from build123d import *

# Parameters (mm, degrees)
SZKIC2_W                    = 70
SZKIC2_H                    = 50
DODANIE_WYCI_GNI_CIE1_DEPTH = 5
OTW_R_3_2_3_2_1_D           = 3.2
OTW_R_3_2_3_2_1_DEPTH       = 5
OTW_R_3_2_3_2_1_TIP         = 0.96137699
WYTNIJ_WYCI_GNI_CIE1_REACH  = 45.301
SZKIC7_R                    = 6
DODANIE_WYCI_GNI_CIE2_DEPTH = 5
SFAZOWANIE1_SIZE            = 2


with BuildPart() as part:
    # Szkic2 → Dodanie-wyciągnięcie1 (new body)
    with BuildSketch(Plane(origin=(0, 0, 0), x_dir=(1, 0, 0), z_dir=(0, 1, 0))):
        Rectangle(SZKIC2_W, SZKIC2_H)
    extrude(amount=DODANIE_WYCI_GNI_CIE1_DEPTH)

    # Otwór Ø3.2 (3.2)1
    with Locations(Plane(origin=(0, 5, 0), x_dir=(1, 0, 0), z_dir=(0, 1, 0))):
        with Locations((-7.75, -14.423393759), (7.75, -14.423393759), (15.5, -1), (7.75, 12.423393759), (-7.75, 12.423393759), (-15.5, -1)):
            Hole(OTW_R_3_2_3_2_1_D / 2, depth=OTW_R_3_2_3_2_1_DEPTH)
            with Locations((0, 0, -(OTW_R_3_2_3_2_1_DEPTH + OTW_R_3_2_3_2_1_TIP / 2))):  # 118° drill point
                Cone(0, OTW_R_3_2_3_2_1_D / 2, OTW_R_3_2_3_2_1_TIP, mode=Mode.SUBTRACT)

    # Szkic7 → Wytnij-wyciągnięcie1 (cut, up to next)
    with BuildSketch(Plane(origin=(0, 5, 0), x_dir=(1, 0, 0), z_dir=(0, 1, 0)), mode=Mode.PRIVATE) as wytnij_wyci_gni_cie1_sk1:
        with Locations(Location((0, 6, 0), (0, 0, 270))):
            Circle(SZKIC7_R)
    wytnij_wyci_gni_cie1_tool1 = extrude(wytnij_wyci_gni_cie1_sk1.sketch, amount=-WYTNIJ_WYCI_GNI_CIE1_REACH, mode=Mode.PRIVATE) & part.part
    add(wytnij_wyci_gni_cie1_tool1.solids().sort_by_distance((0, 5, -6))[0], mode=Mode.SUBTRACT)

    # Szkic8 → Dodanie-wyciągnięcie2 (add)
    with BuildSketch(Plane(origin=(0, 0, -25), x_dir=(-1, 0, 0), z_dir=(0, 0, -1))):
        Polygon((-35, 5), (-35, 55), (35, 55), (35, 5), (35, 0), (-35, 0), align=None)
    extrude(amount=DODANIE_WYCI_GNI_CIE2_DEPTH)

    # Sfazowanie1
    sfazowanie1_edges = [part.edges().sort_by_distance(p)[0] for p in [
        (0, 5, -25),
    ]]
    chamfer(sfazowanie1_edges, length=SFAZOWANIE1_SIZE)


solid = part.part
Input: part model. Units: mm. Frame: model coordinates. A direction names the side the tool comes from. Give positions to 0.01 mm unless a question says otherwise; leave off trailing zeros. Write each loop counter-clockwise with the first axis right and the second up, starting at its lowest first coordinate (ties: lowest second). Pieces come first, ordered by that corner, then holes. Notation, with made-up numbers: M -33,-14.5 L 17,-14.5 A18 ccw 17,13.5 Z; hole C -24.75,-2.5 d1. An arc over 180 degrees is marked long. Write item = value, one per line. Start each with the question number.
1) Draft query along Z for faces 3 (the flat face through (0, 2, 25)), 4 (the cylindrical face through (7.96, 2.46, -14.01)), 5 (the flat face through (35, 15, -27)). Return one class per face: +Z half, -Z half, draft (parallel to the pull), parting line (faces both ways), or undercut.
2) First-contact query: pin 1 Ø1.9 at (x, z) = (-7.75, -12.42) entering from +Y; pin 2 Ø14.5 at (x, z) = (-16, 3) entering from +Y. Flat tips, straight axial feed; report the tip coordinate or a pass-through.
3) Cut plane C-C on x = -15.5. Return the cut outline in (y, z), then the cut area to 3 significant figures.
4) Cut plane B-B on x = -7.75. Return the cut outline in (y, z).
5) Cut plane D-D on z = -6. Return the cut outline in (x, y), then the cut area to 3 significant figures.
6) Cut plane A-A on z = 1. Return the cut outline in (x, y), then the cut area to 3 significant figures.
7) Reachability of faces 1 (the flat face through (0, 5, 1)), 2 (the cylindrical face through (17.1, 2.46, 0.93)) from +Z, -Z, +X, -X, +Y, -Y: full face, straight path, thin tool, end or side. Return the list, or none.
8) Material intervals for line 1 along Z through (x, y) = (7, 3); line 2 along Z through (x, y) = (-17.5, 9); line 3 along Y through (x, z) = (14, -1), sorted ascending. Write a range as [from, to].
Solved:
q1.face_3 = +Z half
q1.face_4 = undercut
q1.face_5 = draft
q2.pin_1 = through
q2.pin_2 = 5
q3.outline = M 0,-30 L 55,-30 L 55,-25 L 7,-25 L 5,-23 L 5,-0.6 L 0,-0.6 Z; M 0,2.6 L 5,2.6 L 5,25 L 0,25 Z
q3.area = 511 mm2
q4.outline = M 0,-30 L 55,-30 L 55,-25 L 7,-25 L 5,-23 L 5,-14.02 L 0,-14.02 Z; M 0,-10.82 L 5,-10.82 L 5,12.82 L 0,12.82 Z; M 0,16.02 L 5,16.02 L 5,25 L 0,25 Z
q5.outline = M -35,0 L -6,0 L -6,5 L -35,5 Z; M 6,0 L 35,0 L 35,5 L 6,5 Z
q5.area = 290 mm2
q6.outline = M -35,0 L -17.1,0 L -17.1,5 L -35,5 Z; M -13.9,0 L 13.9,0 L 13.9,5 L -13.9,5 Z; M 17.1,0 L 35,0 L 35,5 L 17.1,5 Z
q6.area = 318 mm2
q7.face_1 = +Z, +X, -X, +Y
q7.face_2 = +Y, -Y
q8.line_1 = [-30, -13.84], [-11.01, 13.01], [15.84, 25]
q8.line_2 = [-30, -25]
q8.line_3 = [0, 5]
